Geometry check sheet. Reference: the model listing, model coordinates, mm. Face numbers are marked on the shaded views. A direction names the side the tool comes from. Round coordinates to 2 decimals unless told otherwise and drop trailing zeros. Write each loop counter-clockwise with the first axis right and the second up, starting at its lowest first coordinate (ties: lowest second). Pieces come first, ordered by that corner, then holes.
Item 1: Depth check by flat-ended pin: P1, Ø1.8, axis at y = -13.5, z = 0, coming from the -X side; P2, Ø1.8, axis at x = 0, z = -0.5, coming from the -Y side; P3, Ø2, axis at x = -6.5, z = 0.5, coming from the +Y side; P4, Ø14.5, axis at x = 0, y = 0, coming from the -Z side. Enter the tip coordinate at first touch or a pass-through.
Item 2: Cross-section at B-B (x = 3). Enter the section's corners in (y, z).
Item 3: Cross-section at C-C (y = -15). Enter the section's corners in (x, z).
Item 4: Cross-section at D-D (y = -10). Enter the section's corners in (x, z), then the cut area to 3 significant figures.
Item 5: Draft check along Y on the marked faces 3 and 4. Enter one of: pulls with the +Y half, pulls with the -Y half, needs draft (parallel to the pull), parting line crosses it, or undercut.
Item 6: Scan lines: probe 1 along Y at (x, z) = (0, 0); probe 2 along X at (y, z) = (5, 1.25); probe 3 along X at (y, z) = (8, -1.35). Record each from-to range of solid material in increasing order.
Item 7: Cross-section at A-A (y = 0). Enter the section's corners in (x, z), then the cut area to 3 significant figures.
Item 8: Access from +Z, -Z, +X, -X, +Y, -Y to the whole of each face (thin tool, end or side, straight path). Record for the marked faces 1 and 2.
Autodesk Inventor part; units mm, degrees
ref_plane "YZ Plane" through (0, 0, 0) normal (1, 0, 0) x (0, 1, 0)
ref_plane "XZ Plane" through (0, 0, 0) normal (0, 1, 0) x (-1, 0, 0)
ref_plane "XY Plane" through (0, 0, 0) normal (0, 0, 1) x (1, 0, 0)
sketch "Sketch1" plane through (0, 0, 0) normal (0, 0, 1) x (1, 0, 0)
  circle A0 centre (0, 0) radius 11
  circle A1 centre (0, 0) radius 17
  line L0 (11, 1.75) -> (17, 1.75)
  line L1 (17, 1.75) -> (17, -1.75)
  line L2 (17, -1.75) -> (11, -1.75)
  line L3 (11, -1.75) -> (11, 1.75)
  line L4 (13.2583, 10.7834) -> (9.0156, 6.5407)
  line L5 (9.0156, 6.5407) -> (6.5407, 9.0156)
  line L6 (6.5407, 9.0156) -> (10.7834, 13.2583)
  line L7 (10.7834, 13.2583) -> (13.2583, 10.7834)
  line L8 (1.75, 17) -> (1.75, 11)
  line L9 (1.75, 11) -> (-1.75, 11)
  line L10 (-1.75, 11) -> (-1.75, 17)
  line L11 (-1.75, 17) -> (1.75, 17)
  line L12 (-10.7834, 13.2583) -> (-6.5407, 9.0156)
  line L13 (-6.5407, 9.0156) -> (-9.0156, 6.5407)
  line L14 (-9.0156, 6.5407) -> (-13.2583, 10.7834)
  line L15 (-13.2583, 10.7834) -> (-10.7834, 13.2583)
  line L16 (-17, 1.75) -> (-11, 1.75)
  line L17 (-11, 1.75) -> (-11, -1.75)
  line L18 (-11, -1.75) -> (-17, -1.75)
  line L19 (-17, -1.75) -> (-17, 1.75)
  line L20 (-13.2583, -10.7834) -> (-9.0156, -6.5407)
  line L21 (-9.0156, -6.5407) -> (-6.5407, -9.0156)
  line L22 (-6.5407, -9.0156) -> (-10.7834, -13.2583)
  line L23 (-10.7834, -13.2583) -> (-13.2583, -10.7834)
  line L24 (-1.75, -17) -> (-1.75, -11)
  line L25 (-1.75, -11) -> (1.75, -11)
  line L26 (1.75, -11) -> (1.75, -17)
  line L27 (1.75, -17) -> (-1.75, -17)
  line L28 (10.7834, -13.2583) -> (6.5407, -9.0156)
  line L29 (6.5407, -9.0156) -> (9.0156, -6.5407)
  line L30 (9.0156, -6.5407) -> (13.2583, -10.7834)
  line L31 (13.2583, -10.7834) -> (10.7834, -13.2583)
  circle A2 centre (0, 0) radius 9
  circle A3 centre (0, 0) radius 19
  line L32 (-13.035, -5.3993) -> (-5.3993, 13.035)
  line L33 (-5.3993, 13.035) -> (13.035, 5.3993)
  line L34 (13.035, 5.3993) -> (5.3993, -13.035)
  line L35 (5.3993, -13.035) -> (-13.035, -5.3993)
  line L36 (0, 0) -> (-5.3993, 13.035)
  line L37 (0, 0) -> (14.109, 0) construction
  line L38 (0, 0) -> (16.0476, 6.6471)
  line L39 (0, 0) -> (17.3698, 0) construction
  circle A4 centre (-5.3993, 13.035) radius 0.5
  circle A5 centre (13.035, 5.3993) radius 0.5
  circle A6 centre (5.3993, -13.035) radius 0.5
  circle A7 centre (-13.035, -5.3993) radius 0.5
  point P0 (11, 0)
  point P1 (7.7782, 7.7782)
  point P2 (0, 11)
  point P3 (-7.7782, 7.7782)
  point P4 (-11, 0)
  point P5 (-7.7782, -7.7782)
  point P6 (0, -11)
  point P7 (7.7782, -7.7782)
  dimension "d0" = 22
  dimension "d1" = 6
  dimension "d2" = 3.5
  dimension "d3" = 6
  dimension "d6" = 360
  dimension "d8" = 2
  dimension "d9" = 2
  dimension "d23" = 112.5
  dimension "d24" = 22.5
  dimension "d25" = 1
  dimension "d26" = 1
  dimension "d27" = 1
  dimension "d28" = 1
  dimension "d29" = 14.109
  dimension "d30" = 19.9531
  dimension "d31" = 19.9531
extrude "Extrusion1" add sketch "Sketch1" along normal mid plane 3.5 contours A0 L34 | L3 L2 A1 L30 L29 A0 | A0 L34 L3 | L34 A0 L35 L32 L36 A2 L38 | A0 L38 A5 L34 L0 L3 | L29 L34 A0 | L38 A2 L36 A0 L33 | A0 L33 L5 L4 A5 L38 | L34 L29 L28 A6 L35 L26 L25 A0 | L34 A5 L38 A1 L0 | L33 A0 | A0 L5 L33 | L35 L25 A0 | A0 L35 | L28 A1 L26 L35 A6 L34 | A0 L9 L8 A1 L6 L5 | L33 L9 A0 | A0 L36 A4 L33 L10 L9 | L33 L4 A1 L38 A5 | L25 L24 A1 L22 L21 A0 | L35 L21 L20 A7 L32 L18 L17 A0 | A0 L21 L35 | A0 L32 L13 L12 A4 L36 | L32 L17 A0 | A0 L32 | A0 L13 L32 | L33 A4 L32 L12 A1 L10 | L17 L16 A1 L14 L13 A0 | L20 A1 L18 L32 A7 L35 | A3
equation "\"d25\" = d28"
equation "\"d26\" = d28"
equation "\"d27\" = d28"
properties part number "Spodnji obroc"
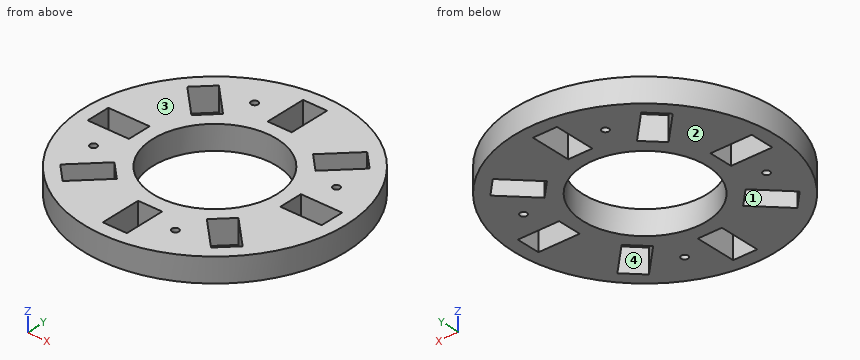
Resolved:
1. P1: stops at x = -14.22
1. P2: stops at y = -19
1. P3: stops at y = 18.19
1. P4: passes through
2. outline: (-18.76, -1.75) - (-8.49, -1.75) - (-8.49, 1.75) - (-18.76, 1.75) - close; (8.49, -1.75) - (18.76, -1.75) - (18.76, 1.75) - (8.49, 1.75) - close
3. outline: (-11.66, -1.75) - (-1.75, -1.75) - (-1.75, 1.75) - (-11.66, 1.75) - close; (1.75, -1.75) - (11.66, -1.75) - (11.66, 1.75) - (1.75, 1.75) - close
4. outline: (-16.16, -1.75) - (-12.47, -1.75) - (-12.47, 1.75) - (-16.16, 1.75) - close; (-7.53, -1.75) - (7.53, -1.75) - (7.53, 1.75) - (-7.53, 1.75) - close; (12.47, -1.75) - (16.16, -1.75) - (16.16, 1.75) - (12.47, 1.75) - close
4. area: 78.4 mm2
5. face 3: needs draft
5. face 4: undercut
6. probe 1: y = -19 to -17, -11 to -9, 9 to 11, 17 to 19
6. probe 2: x = -18.33 to -7.48, 7.48 to 12.73, 13.34 to 18.33
6. probe 3: x = -17.23 to -10.47, -7.56 to -4.12, 4.12 to 7.56, 10.47 to 17.23
7. outline: (-19, -1.75) - (-17, -1.75) - (-17, 1.75) - (-19, 1.75) - close; (-11, -1.75) - (-9, -1.75) - (-9, 1.75) - (-11, 1.75) - close; (9, -1.75) - (11, -1.75) - (11, 1.75) - (9, 1.75) - close; (17, -1.75) - (19, -1.75) - (19, 1.75) - (17, 1.75) - close
7. area: 28.0 mm2
8. face 1: +Z, -Z
8. face 2: -Z, +X, -X, +Y, -Y
